The listing builds one solid part. Answer for the finished solid, in the listing's coordinates (mm). Round coordinates to 2 decimals unless told otherwise and drop trailing zeros. Loops run counter-clockwise (first coordinate to the right, second up) from the corner with the lowest first, then second, coordinate; pieces in that order, holes last. Notation, with made-up numbers: (-14, 12) - (22, 12) arc R20 cw to (22, 38) - close; hole circle Ø2 at (53, 7). An arc over 180 degrees is marked (long way). One line per item, written item: value.
```python
from build123d import *

# Parameters (mm, degrees)
BOSS_EXTRUDE1_DEPTH = 1.25
SKETCH2_W           = 0.5
SKETCH2_H           = 0.5
CUT_EXTRUDE1_DEPTH  = 3.5


with BuildPart() as part:
    # Sketch1 → Boss-Extrude1 (new body, symmetric)
    with BuildSketch(Plane(origin=(0, 0, 0), x_dir=(1, 0, 0), z_dir=(0, 1, 0))):
        Polygon((-0.775, 1.275), (-1.275, 0.775), (-1.275, -0.775), (-0.775, -1.275), (0.775, -1.275), (1.275, -0.775), (1.775, -1.275), (3.325, -1.275), (3.825, -0.775), (4.325, -1.275), (5.875, -1.275), (6.375, -0.775), (6.875, -1.275), (8.425, -1.275), (8.925, -0.775), (9.425, -1.275), (10.975, -1.275), (11.475, -0.775), (11.975, -1.275), (13.525, -1.275), (14.025, -0.775), (14.025, 0.775), (13.525, 1.275), (11.975, 1.275), (11.475, 0.775), (10.975, 1.275), (9.425, 1.275), (8.925, 0.775), (8.425, 1.275), (6.875, 1.275), (6.375, 0.775), (5.875, 1.275), (4.325, 1.275), (3.825, 0.775), (3.325, 1.275), (1.775, 1.275), (1.275, 0.775), (0.775, 1.275), align=None)
    extrude(amount=BOSS_EXTRUDE1_DEPTH, both=True)

    # Sketch2 → Cut-Extrude1 (cut, through all)
    with BuildSketch(Plane(origin=(0, 1.25, 0), x_dir=(1, 0, 0), z_dir=(0, 1, 0))):
        with Locations((2.55, 0)):
            Rectangle(SKETCH2_W, SKETCH2_H)
        Rectangle(SKETCH2_W, SKETCH2_H)
        with Locations((5.1, 0)):
            Rectangle(SKETCH2_W, SKETCH2_H)
        with Locations((7.65, 0)):
            Rectangle(SKETCH2_W, SKETCH2_H)
        with Locations((10.2, 0)):
            Rectangle(SKETCH2_W, SKETCH2_H)
        with Locations((12.75, 0)):
            Rectangle(SKETCH2_W, SKETCH2_H)
    extrude(amount=-CUT_EXTRUDE1_DEPTH, mode=Mode.SUBTRACT)


solid = part.part
```
1) Consider L1, parallel to X at y = 0.5, z = 1.1; L2, parallel to X at y = 0.45, z = 1.2; L3, parallel to Z at x = 11, y = 0.4. Determine where each line is inside the solid, lowest interval first.
Final values:
L1: -0.95 to 0.95, 1.6 to 3.5, 4.15 to 6.05, 6.7 to 8.6, 9.25 to 11.15, 11.8 to 13.7
L2: -0.85 to 0.85, 1.7 to 3.4, 4.25 to 5.95, 6.8 to 8.5, 9.35 to 11.05, 11.9 to 13.6
L3: -1.25 to 1.25
2) A cutting plane is placed at C-C on y = 1.05. Give the number of separate pieces and of enclosed holes in the cut face, and give its area (3 significant figures).
Final values:
separate pieces: 1
enclosed holes: 6
area: 34.5 mm2
3) A cutting plane is placed at B-B on z = 0.05. Give the vertices of the cut face in (x, y) (3 decimals).
Final values:
outline: (-1.275, -1.25) - (-0.25, -1.25) - (-0.25, 1.25) - (-1.275, 1.25) - close; (0.25, -1.25) - (2.3, -1.25) - (2.3, 1.25) - (0.25, 1.25) - close; (2.8, -1.25) - (4.85, -1.25) - (4.85, 1.25) - (2.8, 1.25) - close; (5.35, -1.25) - (7.4, -1.25) - (7.4, 1.25) - (5.35, 1.25) - close; (7.9, -1.25) - (9.95, -1.25) - (9.95, 1.25) - (7.9, 1.25) - close; (10.45, -1.25) - (12.5, -1.25) - (12.5, 1.25) - (10.45, 1.25) - close; (13, -1.25) - (14.025, -1.25) - (14.025, 1.25) - (13, 1.25) - close
4) A cutting plane is placed at A-A on x = 12.75. Give the vertices of the cut face in (y, z) (3 decimals), and give its area (4 significant figures).
Final values:
outline: (-1.25, -1.275) - (1.25, -1.275) - (1.25, -0.25) - (-1.25, -0.25) - close; (-1.25, 0.25) - (1.25, 0.25) - (1.25, 1.275) - (-1.25, 1.275) - close
area: 5.125 mm2
5) A cutting plane is placed at D-D on x = 3.5. Give the vertices of the cut face in (y, z).
Final values:
outline: (-1.25, -1.1) - (1.25, -1.1) - (1.25, 1.1) - (-1.25, 1.1) - close
